from build123d import *

# Parameters (mm, degrees)
CROQUIS1_W              = 52
CROQUIS1_H              = 40
SALIENTE_EXTRUIR1_DEPTH = 3
CROQUIS2_W              = 6
CROQUIS2_H              = 15
CORTAR_EXTRUIR1_DEPTH   = 34.346664001
CORTAR_EXTRUIR2_DEPTH   = 34.346664001


with BuildPart() as part:
    # Croquis1 → Saliente-Extruir1 (new, symmetric)
    with BuildSketch(Plane(origin=(0, 0, 0), x_dir=(1, 0, 0), z_dir=(0, 1, 0))):
        Rectangle(CROQUIS1_W, CROQUIS1_H)
    extrude(amount=SALIENTE_EXTRUIR1_DEPTH, both=True)

    # Croquis2 → Cortar-Extruir1 (cut, through all)
    with BuildSketch(Plane(origin=(0, 3, 0), x_dir=(1, 0, 0), z_dir=(0, 1, 0))):
        with Locations((-20.51875, 0)):
            Rectangle(CROQUIS2_W, CROQUIS2_H)
        with Locations((20.51875, 0)):
            Rectangle(CROQUIS2_W, CROQUIS2_H)
    extrude(amount=-CORTAR_EXTRUIR1_DEPTH, mode=Mode.SUBTRACT)

    # Croquis3 → Cortar-Extruir2 (cut, through all)
    with BuildSketch(Plane(origin=(0, 3, 0), x_dir=(1, 0, 0), z_dir=(0, 1, 0))):
        with BuildLine():
            ThreePointArc((3.403388834, -1.433333333), (0, 12.75), (-3.403388834, -1.433333333))
            ThreePointArc((-3.403388834, -1.433333333), (0, -5.75), (3.403388834, -1.433333333))
        make_face()
    extrude(amount=-CORTAR_EXTRUIR2_DEPTH, mode=Mode.SUBTRACT)


solid = part.part
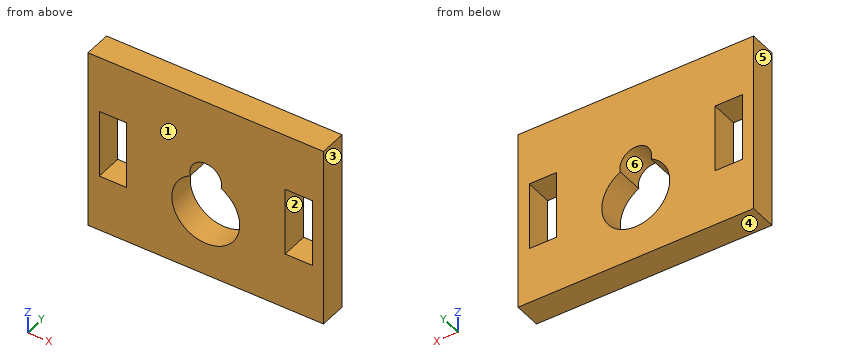
Read the model definition and answer for the solid it produces. Units are mm, in the model's axes. Face numbers are marked on the shaded views. A direction names the side the tool comes from. Coordinates: 2 decimals unless noted, no trailing zeros. Loops run counter-clockwise (first coordinate to the right, second up) from the corner with the lowest first, then second, coordinate; pieces in that order, holes last. Notation, with made-up numbers: (-28, -27) -> (-4, -27) arc R16 cw to (-4, -9) -> close; hole circle Ø9 at (49.5, 26). An arc over 180 degrees is marked (long way). Answer in a Markdown table with one row per item.
Item 1: A cutting plane is placed at C-C on z = 2.25. Determine the outline of the cut face in (x, y), plus the area to 3 significant figures.
Returned:
| item | result |
|---|---|
| outline | (-26, -3) -> (-23.52, -3) -> (-23.52, 3) -> (-26, 3) -> close; (-17.52, -3) -> (-3.5, -3) -> (-3.5, 3) -> (-17.52, 3) -> close; (3.5, -3) -> (17.52, -3) -> (17.52, 3) -> (3.5, 3) -> close; (23.52, -3) -> (26, -3) -> (26, 3) -> (23.52, 3) -> close |
| area | 198 mm^2 |
Item 2: A cutting plane is placed at B-B on z = -5.25. Determine the outline of the cut face in (x, y).
Returned:
| item | result |
|---|---|
| outline | (-26, -3) -> (-23.52, -3) -> (-23.52, 3) -> (-26, 3) -> close; (-17.52, -3) -> (-7.5, -3) -> (-7.5, 3) -> (-17.52, 3) -> close; (7.5, -3) -> (17.52, -3) -> (17.52, 3) -> (7.5, 3) -> close; (23.52, -3) -> (26, -3) -> (26, 3) -> (23.52, 3) -> close |
Item 3: A cutting plane is placed at D-D on y = 0.9. Determine the outline of the cut face in (x, z), plus the area to 3 significant figures.
Returned:
| item | result |
|---|---|
| outline | (-26, -20) -> (26, -20) -> (26, 20) -> (-26, 20) -> close; hole (-23.52, -7.5) -> (-17.52, -7.5) -> (-17.52, 7.5) -> (-23.52, 7.5) -> close; hole (-3.4, 1.43) arc R7.5 ccw (long way) to (3.4, 1.43) arc R3.5 ccw (long way) to start; hole (17.52, -7.5) -> (23.52, -7.5) -> (23.52, 7.5) -> (17.52, 7.5) -> close |
| area | 1,700 mm^2 |
Item 4: This flat-tipped pin is pushed along its axis until it touches: P1, Ø12, axis at x = 0, z = -5.25, coming from the +Y side. Where does it stop, or does it pass through?
Returned:
| item | result |
|---|---|
| P1 | passes through |
Item 5: For the marked faces 1 and 2, determine the directions among +Z, -Z, +X, -X, +Y, -Y from which every point of the face is accessible in a straight line to the end or side of a thin tool.
Returned:
| item | result |
|---|---|
| face 1 | +Z, -Z, +X, -X, -Y |
| face 2 | +Y, -Y |
Item 6: A cutting plane is placed at A-A on x = -20.5. Determine the outline of the cut face in (y, z).
Returned:
| item | result |
|---|---|
| outline | (-3, -20) -> (3, -20) -> (3, -7.5) -> (-3, -7.5) -> close; (-3, 7.5) -> (3, 7.5) -> (3, 20) -> (-3, 20) -> close |
Item 7: Straight lines are drawn through the part: line 1 along X through (y, z) = (-0.95, -5.25); line 2 along X through (y, z) = (1, 2.25); line 3 along Z through (x, y) = (-18.5, -1.6). For each, find the intervals that lie inside material, in ascending order. Write a range as [from, to].
Returned:
| item | result |
|---|---|
| line 1 | x = [-26, -23.52], [-17.52, -7.5], [7.5, 17.52], [23.52, 26] |
| line 2 | x = [-26, -23.52], [-17.52, -3.5], [3.5, 17.52], [23.52, 26] |
| line 3 | z = [-20, -7.5], [7.5, 20] |
Item 8: For a pull along X with two mould halves and no side action, classify the marked faces 3, 4, 5 and 6 as released by +X, released by -X, zero draft, split by the parting line, or undercut.
Returned:
| item | result |
|---|---|
| face 3 | released by +X |
| face 4 | zero draft |
| face 5 | released by -X |
| face 6 | undercut |
